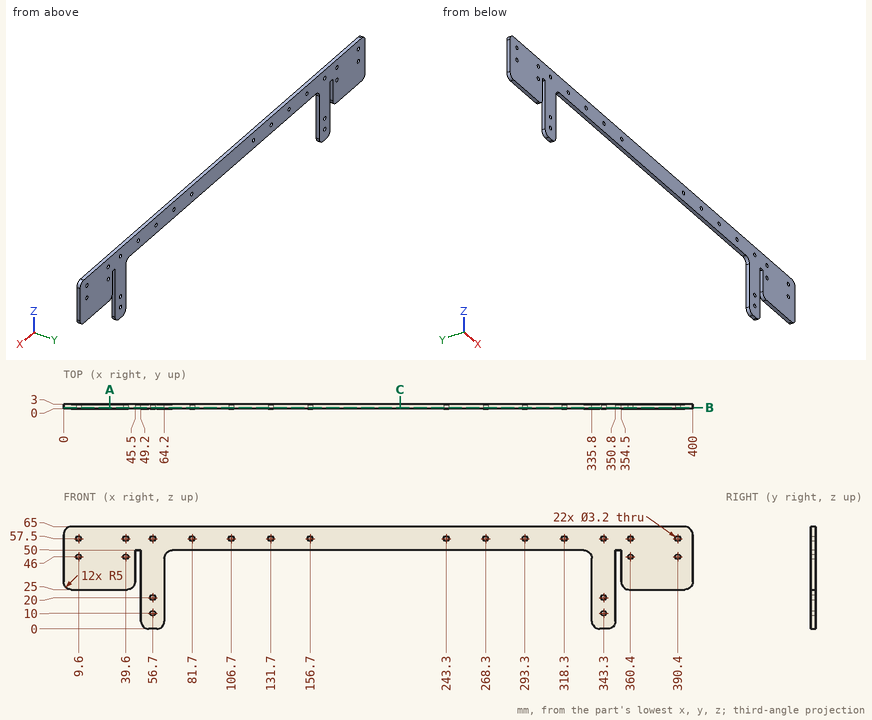
Could you check a few things on this drawing? It's one solid part, dimensions in mm from its lowest x, y, z. Coordinates: 2 decimals unless noted, no trailing zeros. Write each loop counter-clockwise with the first axis right and the second up, starting at its lowest first coordinate (ties: lowest second). Pieces come first, ordered by that corner, then holes. Notation, with made-up numbers: M 34,-24.5 L 50,-24.5 A19 ccw 50,10.5 Z; hole C 55,80.5 d11. An arc over 180 degrees is marked long. One line per question, with ' | ' between items.
1) Imagine slicing it at A-A, the plane x = 29.5. Write out the boundary of the cut face in (y, z).
Checks:
outline: M 0,25 L 3,25 L 3,65 L 0,65 Z
2) Imagine slicing it at C-C, the plane x = 214. Write out the boundary of the cut face in (y, z).
Checks:
outline: M 0,50 L 3,50 L 3,65 L 0,65 Z
3) I need wall thicknesses on probe 1 along X at (y, z) = (1.25, 40); probe 2 along Z at (x, y) = (360.4, 1); probe 3 along X at (y, z) = (1.55, 12). Which ranges of each line are inside material? Lowest first, please. Write a range as [from, to].
Checks:
probe 1: [0, 45.5], [49.2, 64.2], [335.8, 350.8], [354.5, 400] | probe 2: [25, 44.4], [47.6, 55.9], [59.1, 65] | probe 3: [49.2, 64.2], [335.8, 350.8]
4) For pin 1 Ø1.5 at (x, y) = (17.5, 1) entering from -Z; pin 2 Ø5 at (x, z) = (56.7, 20) entering from -Y; pin 3 Ø1.5 at (x, y) = (143.5, 1.5) entering from -Z, each with a flat end and sliding along its axis, tell me the tip position at first contact or that it passes through.
Checks:
pin 1: z = 25 | pin 2: y = 0 | pin 3: z = 50
5) Imagine slicing it at B-B, the plane y = 0.65. Give the number of separate pieces and of enclosed holes in the cut face, and give its area (3 significant figures).
Checks:
separate pieces: 1 | enclosed holes: 22 | area: 9,560 mm²
